Check sheet for the modelled part. Datum: model origin and axes. Units: mm. A direction names the side the tool comes from. Round coordinates to 2 decimals unless told otherwise and drop trailing zeros. Loops run counter-clockwise (first coordinate to the right, second up) from the corner with the lowest first, then second, coordinate; pieces in that order, holes last. Notation, with made-up numbers: (83.5, -10.75) -> (132.5, -10.75) arc R23 ccw to (132.5, 10.25) -> close; hole circle Ø1 at (51.5, 28.25). An arc over 180 degrees is marked (long way). One line per item, written item: value. Start each with the question number.
1. Cross-section at A-A on z = 0. Record the cut outline in (x, y), then the cut area to 3 significant figures.
2. Go/stop test with flat-tipped pins: pin 1 (5 mm diameter, centred on x = -30, z = -79.5, fed in from +Y); pin 2 (6 mm diameter, centred on x = -47, y = 58.5, fed in from +Z); pin 3 (8 mm diameter, centred on y = 13, z = 11.5, fed in from -X). Record where each tip stops, or that it passes through.
3. Material ranges on L1, parallel to X at y = 95, z = 0; L2, parallel to Y at x = -18, z = -82; L3, parallel to X at y = 76.5, z = -15.5, recorded low to high.
4. Release check for a two-part mould opening along X. For faces 4 (the face through (-38, 100, 93)), 5 (the face through (-100.063, 70.14, -22.22)), 6 (the face through (31.54, 54.37, 100.15)) record: +X half, -X half, draft (parallel to the pull), parting line (faces both ways), or undercut.
5. Set-up check for faces 1 (the face through (30.04, 90.14, 95.38)), 2 (the face through (1, 0, -1)), 3 (the face through (-98, 80, 22)): record each of +Z, -Z, +X, -X, +Y, -Y from which the full face is reachable in a straight line by a thin tool's end or side.
6. Cross-section at B-B on x = 0. Record the cut outline in (y, z), then the cut area to 3 significant figures.
7. Cross-section at C-C on y = 16. Record the cut outline in (x, z), then the cut area to 3 significant figures.
from build123d import *

# Parameters (mm, degrees)
SKETCH1_R           = 105
BOSS_EXTRUDE2_DEPTH = 100
SKETCH2_R           = 100
CUT_EXTRUDE2_DEPTH  = 50
FILLET1_R           = 10
FILLET2_R           = 10


with BuildPart() as part:
    # Sketch1 → Boss-Extrude2 (new body)
    with BuildSketch(Plane(origin=(0, 0, 0), x_dir=(1, 0, 0), z_dir=(0, 1, 0))):
        with Locations(Location((0, 0, 0), (0, 0, 270))):
            Circle(SKETCH1_R)
    extrude(amount=BOSS_EXTRUDE2_DEPTH)

    # Sketch2 → Cut-Extrude2 (cut)
    with BuildSketch(Plane(origin=(0, 100, 0), x_dir=(1, 0, 0), z_dir=(0, 1, 0))):
        with Locations(Location((0, 0, 0), (0, 0, 270))):
            Circle(SKETCH2_R)
    extrude(amount=-CUT_EXTRUDE2_DEPTH, mode=Mode.SUBTRACT)

    # Fillet1
    fillet1_edges = [part.edges().sort_by_distance(p)[0] for p in [
        (0, 50, -100),
    ]]
    fillet(fillet1_edges, radius=FILLET1_R)

    # Fillet2
    fillet2_edges = [part.edges().sort_by_distance(p)[0] for p in [
        (0, 0, -105),
    ]]
    fillet(fillet2_edges, radius=FILLET2_R)

    # Sketch4 → Cut-Revolve1 (revolve, cut)
    with BuildSketch(Plane.XY, mode=Mode.PRIVATE) as cut_revolve1_sk:
        Polygon((0, 80), (0, 63), (0, 60), (102.5, 60), (102.5, 80), align=None)
    revolve(cut_revolve1_sk.sketch.rotate(Axis((0, 0, 0), (0, 1, 0)), 270), axis=Axis((0, 0, 0), (0, 1, 0)), mode=Mode.SUBTRACT)


solid = part.part
Taken from the geometry:
1. outline: (-105, 10) arc R10 ccw to (-95, 0) -> (95, 0) arc R10 ccw to (105, 10) -> (105, 100) -> (100, 100) -> (100, 80) -> (102.5, 80) -> (102.5, 60) -> (100, 60) arc R10 cw to (90, 50) -> (-90, 50) arc R10 cw to (-100, 60) -> (-102.5, 60) -> (-102.5, 80) -> (-100, 80) -> (-100, 100) -> (-105, 100) -> close
1. area: 10,900 mm2
2. pin 1: stops at y = 50
2. pin 2: stops at z = 95.34
2. pin 3: stops at x = -104.73
3. L1: x = -105 to -100, 100 to 105
3. L2: y = 0 to 50
3. L3: x = -103.85 to -101.32, 101.32 to 103.85
4. face 4: draft
4. face 5: undercut
4. face 6: parting line
5. face 1: +Y
5. face 2: +Z, -Z, +X, -X, -Y
5. face 3: none
6. outline: (0, -95) arc R10 ccw to (10, -105) -> (100, -105) -> (100, -100) -> (80, -100) -> (80, -102.5) -> (60, -102.5) -> (60, -100) arc R10 cw to (50, -90) -> (50, 90) arc R10 cw to (60, 100) -> (60, 102.5) -> (80, 102.5) -> (80, 100) -> (100, 100) -> (100, 105) -> (10, 105) arc R10 ccw to (0, 95) -> close
6. area: 10,900 mm2
7. outline: circle Ø210 at (0, 0)
7. area: 34,600 mm2
